```python
from build123d import *

# Parameters (mm, degrees)
F0_W          = 41.536912322
F0_H          = 86.5394547582
F1_DEPTH      = 12.7
F2_T          = -2.54
F3_R          = 2.2759132083
F5_DEPTH      = 1.524
F4_R          = 2.2733
F6_DEPTH      = 1.524
F7_W          = 7.9097328708
F7_H          = 3.2450191211
F8_DEPTH      = 1.524
F9_R          = 1.27
F10_R         = 5.08
F11_R         = 5.08
F12_T4_DEPTH  = 38.1
F12_T10_DEPTH = 38.1
F12_T16_DEPTH = 38.1
F12_T23_DEPTH = 38.1
F12_T29_DEPTH = 38.1
F13_R         = 5.08
F14_R         = 3.4214532803
F15_DEPTH     = 37.77729
F16_R         = 9.955312615
F17_DEPTH     = 26.73123


# Not quite as in the source:
# - a fillet or chamfer that OpenCascade refuses, or shapes differently, is made with other operations: its cross-section is extruded or revolved along the edge and cut away or added


with BuildPart() as f1:
    # F0 (on Front) → F1 (new body)
    with BuildSketch(Plane.XZ):
        with Locations((-20.768456161, -43.2697273791)):
            Rectangle(F0_W, F0_H)
    extrude(amount=F1_DEPTH)

    # F2
    f2_openings = [f1.faces().sort_by_distance(p)[0] for p in [
        (-20.768456, -12.7, -43.269727),
    ]]
    offset(amount=F2_T, openings=f2_openings)

    # F3 (on face) → F5 (join)
    with BuildSketch(Plane(origin=(-41.536912322, 0, 0), x_dir=(0, -1, 0), z_dir=(-1, 0, 0))):
        with Locations((4.2136539705, -15.7545246184)):
            Circle(F3_R)
    extrude(amount=F5_DEPTH)

    # F4 (on face) → F6 (join)
    with BuildSketch(Plane(origin=(-41.536912322, 0, 0), x_dir=(0, -1, 0), z_dir=(-1, 0, 0))):
        with Locations((3.8371200208, -24.8998850584)):
            Circle(F4_R)
    extrude(amount=F6_DEPTH)

    # F7 (on face) → F8 (join)
    with BuildSketch(Plane.XY):
        with Locations((-8.1125465222, -4.3604943203)):
            Rectangle(F7_W, F7_H)
    extrude(amount=F8_DEPTH)

    # F9
    f9_edges = [f1.edges().sort_by_distance(p)[0] for p in [
        (-8.112547, -2.737985, 1.524),
        (-12.067413, -4.360494, 1.524),
        (-8.112547, -5.983004, 1.524),
        (-4.15768, -4.360494, 1.524),
    ]]
    fillet(f9_edges, radius=F9_R)

    # F10
    f10_edges = [f1.edges().sort_by_distance(p)[0] for p in [
        (-41.536912, -6.35, 0),
    ]]
    fillet(f10_edges, radius=F10_R)

    # F11
    f11_edges = [f1.edges().sort_by_distance(p)[0] for p in [
        (-41.536912, -6.35, -86.539455),
    ]]
    fillet(f11_edges, radius=F11_R)

    # F12: fillet of radius 5.08 on 1 edges, made by hand


with BuildPart() as f12_tool2:
    # F12_s3 → F12_t4 (new body)
    with BuildSketch(Plane.XZ.offset(-12.7)):
        with BuildLine():
            ThreePointArc((-5.08, 0), (-1.4878975516, -1.4878975516), (0, -5.08))
            Line((0, -5.08), (0, 0))
            Line((0, 0), (-5.08, 0))
        make_face()
    extrude(amount=F12_T4_DEPTH)

    split(bisect_by=Plane.YZ.offset(-4.1576800868), keep=Keep.BOTTOM)

    split(bisect_by=Plane.XZ.offset(2.7379847597), keep=Keep.BOTTOM)


with BuildPart() as f1_1:
    add(f1.part)

    # F12_t1: cut F12_tool2
    add(f12_tool2.part, mode=Mode.SUBTRACT)


with BuildPart() as f12_tool8:
    # F12_s9 → F12_t10 (new body)
    with BuildSketch(Plane.XZ.offset(-12.7)):
        with BuildLine():
            ThreePointArc((-5.08, 0), (-1.4878975516, -1.4878975516), (0, -5.08))
            Line((0, -5.08), (0, 0))
            Line((0, 0), (-5.08, 0))
        make_face()
    extrude(amount=F12_T10_DEPTH)

    split(bisect_by=Plane.YZ.offset(-4.1576800868), keep=Keep.TOP)

    split(bisect_by=Plane.XZ.offset(2.7379847597), keep=Keep.BOTTOM)


with BuildPart() as f1_2:
    add(f1_1.part)

    # F12_t7: cut F12_tool8
    add(f12_tool8.part, mode=Mode.SUBTRACT)


with BuildPart() as f12_tool14:
    # F12_s15 → F12_t16 (new body)
    with BuildSketch(Plane.XZ.offset(-12.7)):
        with BuildLine():
            ThreePointArc((-5.08, 0), (-1.4878975516, -1.4878975516), (0, -5.08))
            Line((0, -5.08), (0, 0))
            Line((0, 0), (-5.08, 0))
        make_face()
    extrude(amount=F12_T16_DEPTH)

    split(bisect_by=Plane.YZ.offset(-4.1576800868), keep=Keep.TOP)

    split(bisect_by=Plane.XZ.offset(5.9830038808), keep=Keep.BOTTOM)

    split(bisect_by=Plane.XZ.offset(2.7379847597), keep=Keep.TOP)


with BuildPart() as f1_3:
    add(f1_2.part)

    # F12_t13: cut F12_tool14
    add(f12_tool14.part, mode=Mode.SUBTRACT)


with BuildPart() as f12_tool21:
    # F12_s22 → F12_t23 (new body)
    with BuildSketch(Plane.XZ.offset(-12.7)):
        with BuildLine():
            ThreePointArc((-5.08, 0), (-1.4878975516, -1.4878975516), (0, -5.08))
            Line((0, -5.08), (0, 0))
            Line((0, 0), (-5.08, 0))
        make_face()
    extrude(amount=F12_T23_DEPTH)

    split(bisect_by=Plane.YZ.offset(-4.1576800868), keep=Keep.BOTTOM)

    split(bisect_by=Plane.XZ.offset(5.9830038808), keep=Keep.TOP)


with BuildPart() as f1_4:
    add(f1_3.part)

    # F12_t20: cut F12_tool21
    add(f12_tool21.part, mode=Mode.SUBTRACT)


with BuildPart() as f12_tool27:
    # F12_s28 → F12_t29 (new body)
    with BuildSketch(Plane.XZ.offset(-12.7)):
        with BuildLine():
            ThreePointArc((-5.08, 0), (-1.4878975516, -1.4878975516), (0, -5.08))
            Line((0, -5.08), (0, 0))
            Line((0, 0), (-5.08, 0))
        make_face()
    extrude(amount=F12_T29_DEPTH)

    split(bisect_by=Plane.YZ.offset(-4.1576800868), keep=Keep.TOP)

    split(bisect_by=Plane.XZ.offset(5.9830038808), keep=Keep.TOP)


with BuildPart() as f1_5:
    add(f1_4.part)

    # F12_t26: cut F12_tool27
    add(f12_tool27.part, mode=Mode.SUBTRACT)

    # F13
    f13_edges = [f1_5.edges().sort_by_distance(p)[0] for p in [
        (0, -6.35, -86.539455),
    ]]
    fillet(f13_edges, radius=F13_R)

    # F14 (on face) → F15 (cut)
    with BuildSketch(Plane(origin=(0, 0, 0), x_dir=(-1, 0, 0), z_dir=(0, 1, 0))):
        with Locations((6.212700624, -10.3420317173)):
            Circle(F14_R)
    extrude(amount=-F15_DEPTH, mode=Mode.SUBTRACT)

    # F16 (on face) → F17 (cut)
    with BuildSketch(Plane.XZ.offset(2.54)):
        with Locations((-21.9822023064, -16.7564060539)):
            Circle(F16_R)
    extrude(amount=-F17_DEPTH, mode=Mode.SUBTRACT)


solid = f1_5.part
```
Geometry: final body of the model. Coordinates: model frame, mm. A direction names the side the tool comes from. Coordinates: 2 decimals unless noted, no trailing zeros. Write each loop counter-clockwise with the first axis right and the second up, starting at its lowest first coordinate (ties: lowest second). Pieces come first, ordered by that corner, then holes. Notation, with made-up numbers: M 30.5,-9.5 L 73.5,-9.5 A23 cw 73.5,10.5 Z; hole C -0.75,41 d7. An arc over 180 degrees is marked long. Answer as CSV lines item,"result". Start each with the question number.
Q1. Line query: line 1 (Z direction, x = -26, y = -6.5); line 2 (X direction, y = -4.5, z = -53); line 3 (Z direction, x = -21.5, y = -1). Output: solid intervals per line, ascending. Write a range as from..to.
Q2. Cut plane B-B on z = -9.5. Return the cut outline in (x, y).
Q3. Cut plane C-C on y = -8.25. Return the cut outline in (x, z).
Q4. Pin query (flat end, axial travel): P1, Ø5, axis at y = -3, z = -46, coming from the -X side; P2, Ø5, axis at x = -28.5, y = -7.5, coming from the +Z side; P3, Ø8, axis at x = -27.5, z = -17.5, coming from the -Y side; P4, Ø2, axis at x = -8, z = -23.5, coming from the -Y side. Return the tip coordinate at first contact, or that it passes through.
Q5. Cut plane D-D on x = -21. Return the cut outline in (y, z), then the cut area to 3 significant figures.
Q6. Reachability of faces 4 (the flat face through (-21, -8, -83.999)), 5 (the flat face through (-21, 0, -43)) from +Z, -Z, +X, -X, +Y, -Y: full face, straight path, thin tool, end or side. Return the list, or none.
Q7. Cut plane A-A on x = -33.5. Return the cut outline in (y, z).
Q8. Mould query, pull axis X, two halves, no side actions, for faces 1 (the flat face through (0, -6, -44)), 2 (the cylindrical face through (-42.29, -2.41, -17.14)), 3 (the flat face through (-21, -8, -2.54)). Classes: released by +X, released by -X, zero draft, split by the parting line, or undercut.
Findings below:
1,line 1,"z = -86.54..-84, -2.54..0"
1,line 2,"x = -41.54..-39, -2.54..0"
1,line 3,"z = -86.54..-26.7, -6.81..0"
2,outline,"M -41.54,-12.7 L -39,-12.7 L -39,-2.54 L -28.8,-2.54 L -28.8,0 L -41.54,0 Z; M -15.17,-2.54 L -9.53,-2.54 L -9.53,0 L -15.17,0 Z; M -2.9,-2.54 L -2.54,-2.54 L -2.54,-12.7 L 0,-12.7 L 0,0 L -2.9,0 Z"
3,outline,"M -41.54,-81.46 A5.08 ccw -36.46,-86.54 L -5.08,-86.54 A5.08 ccw 0,-81.46 L 0,-5.08 A5.08 ccw -5.08,0 L -36.46,0 A5.08 ccw -41.54,-5.08 Z; hole M -39,-84 L -2.54,-84 L -2.54,-2.54 L -39,-2.54 Z"
4,P1,"stops at x = -41.54"
4,P2,"stops at z = 0"
4,P3,"passes through"
4,P4,"stops at y = -2.54"
5,outline,"M -12.7,-86.54 L 0,-86.54 L 0,-26.66 L -2.54,-26.66 L -2.54,-84 L -12.7,-84 Z; M -12.7,-2.54 L -2.54,-2.54 L -2.54,-6.85 L 0,-6.85 L 0,0 L -12.7,0 Z"
5,area,"221 mm2"
6,face 4,"-Y"
6,face 5,"+Z, -Z, +X, -X, +Y"
7,outline,"M -12.7,-86.54 L 0,-86.54 L 0,0 L -12.7,0 L -12.7,-2.54 L -2.54,-2.54 L -2.54,-84 L -12.7,-84 Z"
8,face 1,"released by +X"
8,face 2,"zero draft"
8,face 3,"undercut"
